Source: three-view drawing plus pictorial views. Frame: mm from the lowest corner of the part. A direction names the side the tool comes from. Give positions to 0.01 mm unless a question says otherwise; leave off trailing zeros. Loops run counter-clockwise (first coordinate to the right, second up) from the corner with the lowest first, then second, coordinate; pieces in that order, holes last. Notation, with made-up numbers: (64.5, 16.5) -> (99.5, 16.5) arc R17 cw to (99.5, 31.5) -> close; hole circle Ø6 at (-25, 70.5). An arc over 180 degrees is marked (long way). Answer as a JSON object with one key per item and string values. Group by question number.
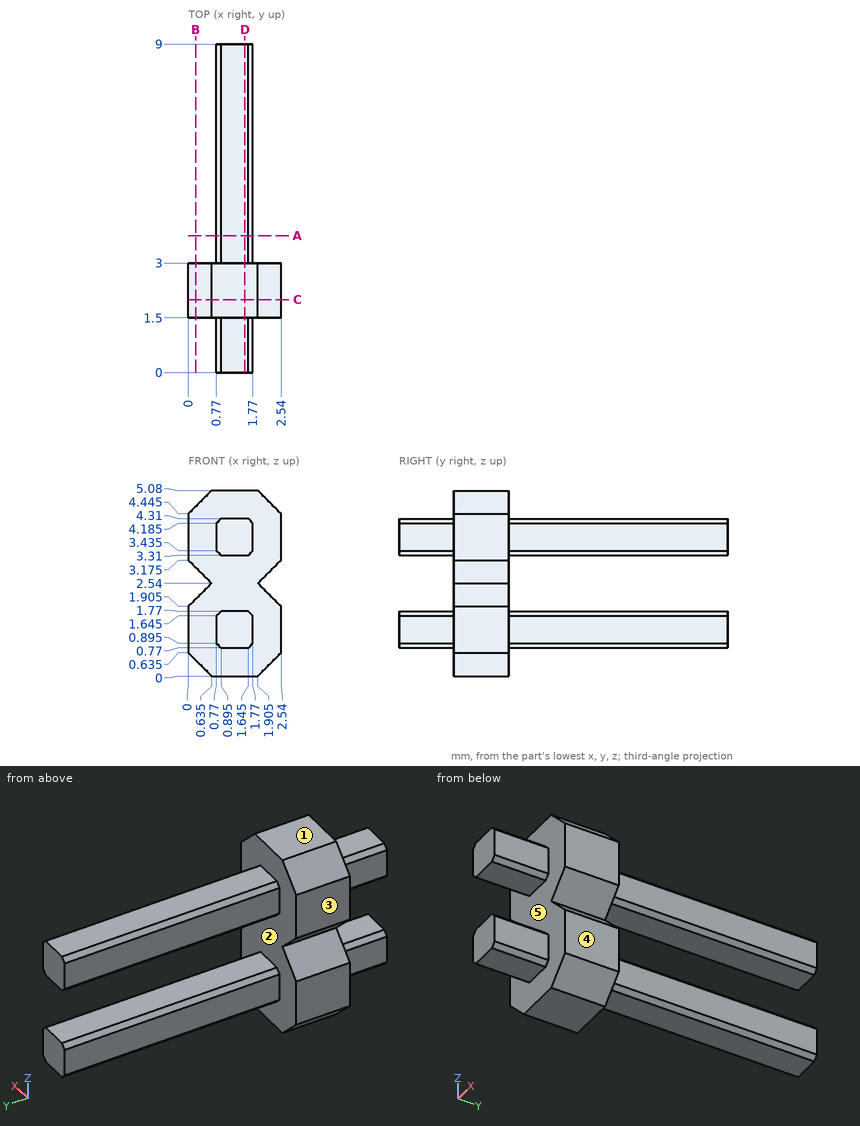
Q1. Section C-C on y = 2. Return the cut outline in (x, z) (3 decimals), then the cut area to 3 significant figures.
Q2. Pin query (flat end, axial travel): pin 1 Ø1 at (x, z) = (1, 3) entering from +Y; pin 2 Ø0.8 at (y, z) = (7.5, 1) entering from +X; pin 3 Ø0.6 at (x, y) = (1.5, 0.5) entering from -Z; pin 4 Ø0.8 at (x, z) = (1.5, 2.5) entering from -Y. Return the tip coordinate at first contact, or that it passes through.
Q3. Pull-direction query (Z, two-part tool) for the marked faces 1, 2 and 3; classes: +Z half, -Z half, draft (parallel to the pull), parting line (faces both ways), or undercut.
Q4. Section A-A on y = 3.75. Return the cut outline in (x, z) (3 decimals).
Q5. Section B-B on x = 0.2. Return the cut outline in (y, z) (3 decimals), then the cut area to 3 significant figures.
Q6. Section D-D on x = 1.55. Return the cut outline in (y, z), then the cut area to 3 significant figures.
Q7. Ray query, probe 1 along Z at (x, y) = (1.6, 8.5); probe 2 along X at (y, z) = (4.75, 3.45); probe 3 along Y at (x, z) = (0.5, 1.1). Return the intervals inside material, ascending.
Q8. Set-up query: the marked faces 4 and 5. Return all of +Z, -Z, +X, -X, +Y, -Y with unobstructed straight access to the full face (end or side cutting, diameter ignored); none if empty.
Numbers:
{
 "1": {"outline": "(0, 0.635) -> (0.635, 0) -> (1.905, 0) -> (2.54, 0.635) -> (2.54, 1.905) -> (1.905, 2.54) -> (2.54, 3.175) -> (2.54, 4.445) -> (1.905, 5.08) -> (0.635, 5.08) -> (0, 4.445) -> (0, 3.175) -> (0.635, 2.54) -> (0, 1.905) -> close", "area": "11.3 mm²"},
 "2": {"pin 1": "stops at y = 9", "pin 2": "stops at x = 1.77", "pin 3": "stops at z = 0.77", "pin 4": "stops at y = 1.5"},
 "3": {"face 1": "+Z half", "face 2": "undercut", "face 3": "draft"},
 "4": {"outline": "(0.77, 0.895) -> (0.895, 0.77) -> (1.645, 0.77) -> (1.77, 0.895) -> (1.77, 1.645) -> (1.645, 1.77) -> (0.895, 1.77) -> (0.77, 1.645) -> close; (0.77, 3.435) -> (0.895, 3.31) -> (1.645, 3.31) -> (1.77, 3.435) -> (1.77, 4.185) -> (1.645, 4.31) -> (0.895, 4.31) -> (0.77, 4.185) -> close"},
 "5": {"outline": "(1.5, 0.435) -> (3, 0.435) -> (3, 2.105) -> (1.5, 2.105) -> close; (1.5, 2.975) -> (3, 2.975) -> (3, 4.645) -> (1.5, 4.645) -> close", "area": "5.01 mm²"},
 "6": {"outline": "(0, 0.77) -> (1.5, 0.77) -> (1.5, 0) -> (3, 0) -> (3, 0.77) -> (9, 0.77) -> (9, 1.77) -> (3, 1.77) -> (3, 3.31) -> (9, 3.31) -> (9, 4.31) -> (3, 4.31) -> (3, 5.08) -> (1.5, 5.08) -> (1.5, 4.31) -> (0, 4.31) -> (0, 3.31) -> (1.5, 3.31) -> (1.5, 1.77) -> (0, 1.77) -> close", "area": "22.6 mm²"},
 "7": {"probe 1": "z = 0.77 to 1.77, 3.31 to 4.31", "probe 2": "x = 0.77 to 1.77", "probe 3": "y = 1.5 to 3"},
 "8": {"face 4": "+Z, -Z, +X, +Y, -Y", "face 5": "-Y"}
}
